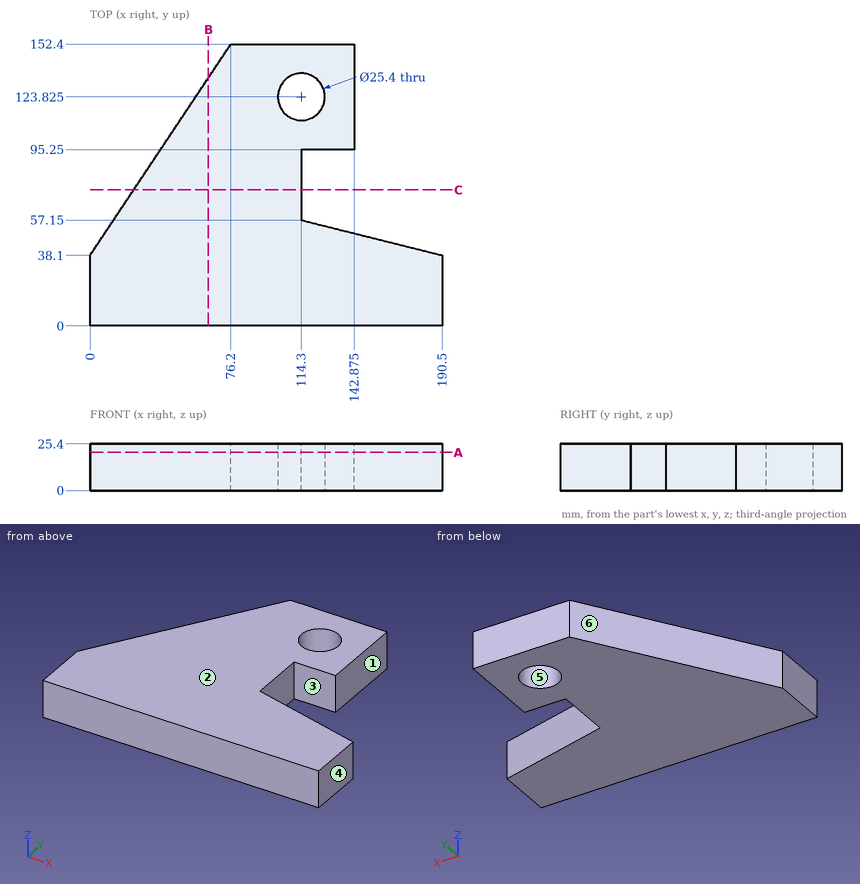
The figure shows three views and two pictorial views of one solid part (mm, origin at its lowest corner). Answer the questions. A direction names the side the tool comes from. Round coordinates to 2 decimals unless told otherwise and drop trailing zeros. Order: outer loops, then holes, each group sorted by start corner. A loop starts at its lowest first (then second) coordinate and runs counter-clockwise, first axis right, second up.
Q1. A cutting plane is placed at C-C, the plane y = 73.5. Determine the outline of the cut face in (x, z), then the cut area to 3 significant figures.
Solution:
outline: (23.6, 0) - (114.3, 0) - (114.3, 25.4) - (23.6, 25.4) - close
area: 2,300 mm2
Q2. A cutting plane is placed at B-B, the plane x = 64. Determine the outline of the cut face in (y, z), then the cut area to 3 significant figures.
Solution:
outline: (0, 0) - (134.1, 0) - (134.1, 25.4) - (0, 25.4) - close
area: 3,410 mm2
Q3. A cutting plane is placed at A-A, the plane z = 20.75. Determine the outline of the cut face in (x, y) (3 decimals), then the cut area to 3 significant figures.
Solution:
outline: (0, 0) - (190.5, 0) - (190.5, 38.1) - (114.3, 57.15) - (114.3, 95.25) - (142.875, 95.25) - (142.875, 152.4) - (76.2, 152.4) - (0, 38.1) - close; hole circle Ø25.4 at (114.3, 123.825)
area: 17,800 mm2
Q4. The mould has two halves that part along X. Classify the marked faces 4, 5 and 6: pulls with the +X half, pulls with the -X half, needs draft (parallel to the pull), parting line crosses it, or undercut.
Solution:
face 4: pulls with the +X half
face 5: undercut
face 6: pulls with the -X half
Q5. Find the intervals of material crossed by line 1 along Y through (x, z) = (124.5, 14.5); line 2 along Y through (x, z) = (103, 6.25); line 3 along Y through (x, z) = (112, 13) (3 decimals), in increasing order.
Solution:
line 1: y = 0 to 54.6, 95.25 to 116.26, 131.39 to 152.4
line 2: y = 0 to 118.03, 129.62 to 152.4
line 3: y = 0 to 111.335, 136.315 to 152.4
Q6. Given pin 1 Ø1 at (y, z) = (106, 5) entering from +X (3 decimals); pin 2 Ø8 at (y, z) = (66, 14) entering from +X; pin 3 Ø2 at (y, z) = (29, 11.5) entering from -X; pin 4 Ø1.5 at (x, z) = (42.5, 13) entering from +Y (3 decimals), each flat-ended and moving along its own axis, determine where each tip first touches the part or whether it passes through.
Solution:
pin 1: stops at x = 142.875
pin 2: stops at x = 114.3
pin 3: stops at x = 0
pin 4: stops at y = 102.975
Q7. A tool of negligible diameter and unlimited length cuts with its end or side. For the marked faces 1, 2 and 3, from which of +Z, -Z, +X, -X, +Y, -Y can it reach the whole face along a straight path? Write none if from no direction.
Solution:
face 1: +Z, -Z, +X, +Y
face 2: +Z, +X, -X, +Y, -Y
face 3: +Z, -Z, +X
